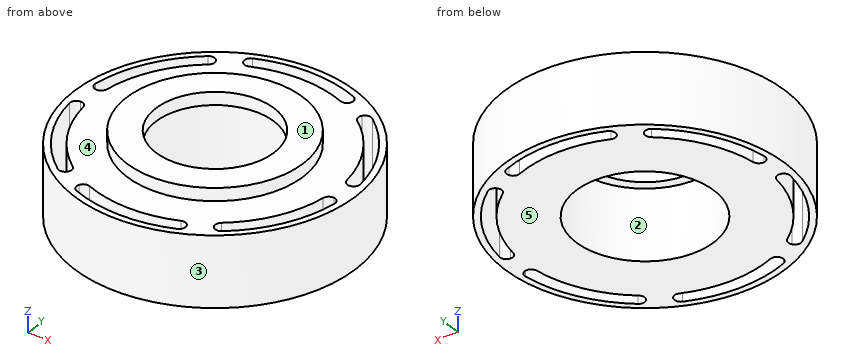
```python
from build123d import *

# Parameters (mm, degrees)
F0_R            = 55.88
F0_R_2          = 27.432
F1_DEPTH        = 27.94
F2_R            = 35.052
F2_R_2          = 23.495
F3_DEPTH        = 5.08
F5_DEPTH        = 27.941
F5_COPIES_COUNT = 6
F6_R            = 2.53999


# Not quite as in the source:
# - a fillet or chamfer is up to 0.001 mm smaller than in the source, because OpenCascade refuses the exact size
# - a pattern or mirror of a feature is missing from the dataset's text; its kind, count and spacing are read off the source's solid


with BuildPart() as f1:
    # F0 (on Top) → F1 (new body)
    with BuildSketch(Plane.XY):
        Circle(F0_R)
        Circle(F0_R_2, mode=Mode.SUBTRACT)
    extrude(amount=F1_DEPTH)

    # F2 (on face) → F3 (join)
    with BuildSketch(Plane.XY.offset(27.94)):
        Circle(F2_R)
        Circle(F2_R_2, mode=Mode.SUBTRACT)
    extrude(amount=F3_DEPTH)

    # F4 (on face) → F5 (cut, through all)
    with BuildSketch(Plane.XY.offset(27.94)):
        with BuildLine():
            ThreePointArc((20.3955573116, -43.7384138024), (0, -48.26), (-20.3955573116, -43.7384138024))
            Line((-20.3955573116, -43.7384138024), (-22.5424580812, -48.3424573605))
            ThreePointArc((-22.5424580812, -48.3424573605), (0, -53.34), (22.5424580812, -48.3424573605))
            Line((22.5424580812, -48.3424573605), (20.3955573116, -43.7384138024))
        make_face()
    f5 = extrude(amount=-F5_DEPTH, mode=Mode.SUBTRACT)

    # F5_copies: F5 ×6 about axis
    f5_copies_axis = Axis((0, 0, 0), (0, 0, 1))
    for i in range(1, F5_COPIES_COUNT):
        add(f5.rotate(f5_copies_axis, i * 360 / F5_COPIES_COUNT), mode=Mode.SUBTRACT)

    # F6 (radius 2.54 in the source; OpenCascade refuses exactly that, so slightly less here)
    f6_edges = [f1.edges().sort_by_distance(p)[0] for p in [
        (-22.542458, -48.342457, 13.97),
        (-20.395557, -43.738414, 13.97),
        (22.542458, -48.342457, 13.97),
        (20.395557, -43.738414, 13.97),
        (-53.137025, -4.648887, 13.97),
        (-48.076356, -4.206136, 13.97),
        (-30.594567, -43.69357, 13.97),
        (-27.680799, -39.532278, 13.97),
        (30.594567, -43.69357, 13.97),
        (27.680799, -39.532278, 13.97),
        (48.076356, -4.206136, 13.97),
        (53.137025, -4.648887, 13.97),
        (-30.594567, 43.69357, 13.97),
        (-27.680799, 39.532278, 13.97),
        (-48.076356, 4.206136, 13.97),
        (-53.137025, 4.648887, 13.97),
        (22.542458, 48.342457, 13.97),
        (20.395557, 43.738414, 13.97),
        (-20.395557, 43.738414, 13.97),
        (-22.542458, 48.342457, 13.97),
        (53.137025, 4.648887, 13.97),
        (48.076356, 4.206136, 13.97),
        (27.680799, 39.532278, 13.97),
        (30.594567, 43.69357, 13.97),
    ]]
    fillet(f6_edges, radius=F6_R)


solid = f1.part
```
Model file for the job. Use its own axes, mm. Face numbers are marked on the shaded views. A direction names the side the tool comes from. Round coordinates to 2 decimals unless told otherwise and drop trailing zeros. Order: outer loops, then holes, each group sorted by start corner. A loop starts at its lowest first (then second) coordinate and runs counter-clockwise, first axis right, second up. Notation, with made-up numbers: (20, 45) -> (56, 45) arc R26 cw to (56, 75) -> close; hole circle Ø3 at (-32, 32.25). An arc over 180 degrees is marked (long way). Use one line per item in the form item = value.
Item 1: Cut at A-A, the plane x = 0. Write the cut outline in (y, z) (3 decimals).
Returned:
outline = (-55.88, 0) -> (-53.34, 0) -> (-53.34, 27.94) -> (-55.88, 27.94) -> close; (-48.26, 0) -> (-27.432, 0) -> (-27.432, 27.94) -> (-23.495, 27.94) -> (-23.495, 33.02) -> (-35.052, 33.02) -> (-35.052, 27.94) -> (-48.26, 27.94) -> close; (23.495, 27.94) -> (27.432, 27.94) -> (27.432, 0) -> (48.26, 0) -> (48.26, 27.94) -> (35.052, 27.94) -> (35.052, 33.02) -> (23.495, 33.02) -> close; (53.34, 0) -> (55.88, 0) -> (55.88, 27.94) -> (53.34, 27.94) -> close
Item 2: Cut at C-C, the plane z = 10.5. Give the number of separate pieces and of enclosed holes in the cut face, and give its area (3 significant figures).
Returned:
separate_pieces = 1
enclosed_holes = 7
area = 6,130 mm^2
Item 3: Flat gauge pins, fed straight in: pin 1 Ø1.5 at (y, z) = (28.5, 10) entering from -X; pin 2 Ø8 at (y, z) = (-36, 24) entering from -X; pin 3 Ø10 at (x, z) = (12.5, 10.5) entering from +Y; pin 4 Ø3 at (x, y) = (10, -27) entering from -Z. Where does each tip first touch, or does it go through?
Returned:
pin_1 = -48.5
pin_2 = -45.81
pin_3 = 55.37
pin_4 = 0
Item 4: Cut at B-B, the plane y = 0. Write the cut outline in (x, z) (3 decimals), and give its area (3 significant figures).
Returned:
outline = (-55.88, 0) -> (-27.432, 0) -> (-27.432, 27.94) -> (-23.495, 27.94) -> (-23.495, 33.02) -> (-35.052, 33.02) -> (-35.052, 27.94) -> (-55.88, 27.94) -> close; (23.495, 27.94) -> (27.432, 27.94) -> (27.432, 0) -> (55.88, 0) -> (55.88, 27.94) -> (35.052, 27.94) -> (35.052, 33.02) -> (23.495, 33.02) -> close
area = 1,710 mm^2
Item 5: Drill centre lines: line 1 (Y direction, x = 0, z = 29) (3 decimals); line 2 (Y direction, x = -9, z = 24); line 3 (Y direction, x = 35, z = 4). Where is each one in solid material? Low to high.
Returned:
line_1 = -35.052 to -23.495, 23.495 to 35.052
line_2 = -55.15 to -52.58, -47.41 to -25.91, 25.91 to 47.41, 52.58 to 55.15
line_3 = -43.56 to -40.25, -33.23 to 33.23, 40.25 to 43.56
Item 6: Pull direction Y, two halves, no side cores. Call the marked faces 1, 2 and 3: released by +Y, released by -Y, zero draft, split by the parting line, or undercut.
Returned:
face_1 = zero draft
face_2 = undercut
face_3 = split by the parting line
Item 7: Tool access for the marked faces 4 and 5: list every direction of +Z, -Z, +X, -X, +Y, -Y with a clear straight run to the whole face (end or side of a thin tool).
Returned:
face_4 = +Z
face_5 = -Z, +X, -X, +Y, -Y
Item 8: Cut at D-D, the plane x = -12. Write the cut outline in (y, z).
Returned:
outline = (-54.58, 0) -> (-51.97, 0) -> (-51.97, 27.94) -> (-54.58, 27.94) -> close; (-46.74, 0) -> (-24.67, 0) -> (-24.67, 27.94) -> (-20.2, 27.94) -> (-20.2, 33.02) -> (-32.93, 33.02) -> (-32.93, 27.94) -> (-46.74, 27.94) -> close; (20.2, 27.94) -> (24.67, 27.94) -> (24.67, 0) -> (46.74, 0) -> (46.74, 27.94) -> (32.93, 27.94) -> (32.93, 33.02) -> (20.2, 33.02) -> close; (51.97, 0) -> (54.58, 0) -> (54.58, 27.94) -> (51.97, 27.94) -> close
